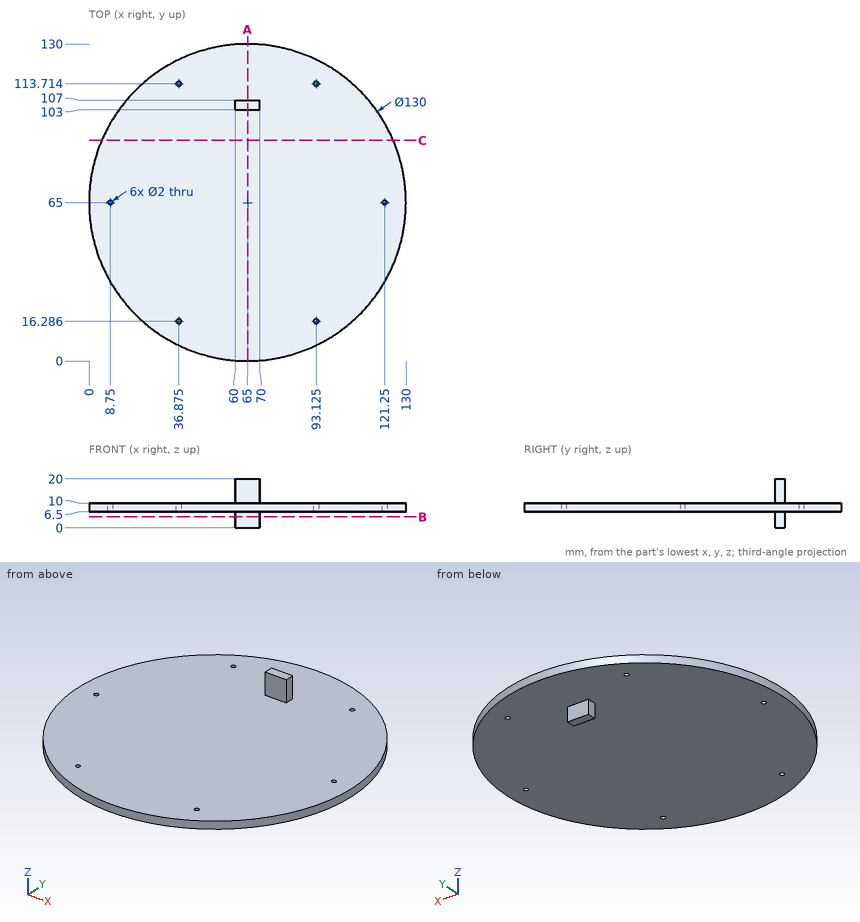
Can you work these out from the drawing? Everything is in mm from the part's minimum corner. Coordinates: 2 decimals unless noted, no trailing zeros. Loops run counter-clockwise (first coordinate to the right, second up) from the corner with the lowest first, then second, coordinate; pieces in that order, holes last. Notation, with made-up numbers: (87.5, 3.25) - (122.5, 3.25) arc R10 cw to (122.5, 17.25) - close; hole circle Ø11 at (6.25, 89.25). An arc over 180 degrees is marked (long way). Put each result on its own line as item: value. Start each with the question number.
Item 1: For pin 1 (2 mm diameter, centred on y = 104.5, z = 14.5, fed in from +X); pin 2 (6 mm diameter, centred on x = 116.5, y = 33.5, fed in from -Z); pin 3 (7 mm diameter, centred on x = 65, z = 3.5, fed in from -Y); pin 4 (1.2 mm diameter, centred on x = 93.12, y = 113.71, fed in from +Z), each with a flat end and sliding along its axis, tell me the tip position at first contact or that it passes through.
Item 2: Suppose I cut it at C-C (y = 90.5). Please give me the cut outline in (x, z).
Item 3: If I drill on line 1 along Z through (x, y) = (108.5, 60); line 2 along Y through (x, z) = (121.25, 7.3); line 3 along Y through (x, z) = (102, 9.25), over which ranges is the centre line in solid material (lowest first)?
Item 4: Suppose I cut it at A-A (x = 65). Please give me the cut outline in (y, z).
Item 5: Suppose I cut it at B-B (z = 4.5). Please give me the cut outline in (x, y).
Here are the results:
1. pin 1: x = 70
1. pin 2: z = 6.5
1. pin 3: y = 0
1. pin 4: through
2. outline: (5.21, 6.5) - (124.79, 6.5) - (124.79, 10) - (5.21, 10) - close
3. line 1: 6.5 to 10
3. line 2: 32.43 to 64, 66 to 97.57
3. line 3: 11.56 to 118.44
4. outline: (0, 6.5) - (103, 6.5) - (103, 0) - (107, 0) - (107, 6.5) - (130, 6.5) - (130, 10) - (107, 10) - (107, 20) - (103, 20) - (103, 10) - (0, 10) - close
5. outline: (60, 103) - (70, 103) - (70, 107) - (60, 107) - close
